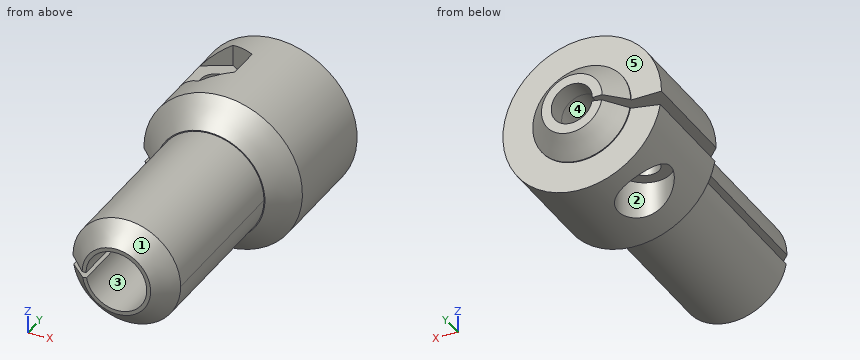
```python
from build123d import *

# Parameters (mm, degrees)
REVOLUTION_ANGLE = 350
SKETCH002_R      = 1.5
POCKET_DEPTH     = 22.101
POCKET001_DEPTH  = 9
SKETCH003_R      = 2.7
POCKET002_DEPTH  = 11
SKETCH004_R      = 8.1
SKETCH004_R_2    = 5.5
POCKET003_DEPTH  = 18
CHAMFER_SIZE     = 2.5
CHAMFER001_SIZE  = 2
PAD_DEPTH        = 2
CHAMFER002_SIZE  = 1.9


with BuildPart() as part:
    # Sketch → Revolution (revolve)
    with BuildSketch(Plane.XY):
        Polygon((-2.1, 8), (-2.1, 0), (-3.1, 0), (-3.1, -23), (-8.1, -23), (-8.1, 8), align=None)
    revolve(axis=Axis((0, 0, 0), (0, 1, 0)), revolution_arc=REVOLUTION_ANGLE)

    # Sketch002 (on DatumPlane) → Pocket (cut, through all)
    with BuildSketch(Plane.XY.offset(14)):
        with Locations((-3.8, 3.2)):
            Circle(SKETCH002_R)
    extrude(amount=-POCKET_DEPTH, mode=Mode.SUBTRACT)

    # Sketch001 (on DatumPlane) → Pocket001 (cut)
    with BuildSketch(Plane.XY.offset(14)):
        Polygon((-3.8, -0.1), (-0.942116, 1.55), (-0.942116, 4.85), (-3.8, 6.5), (-6.657884, 4.85), (-6.657884, 1.55), align=None)
    extrude(amount=-POCKET001_DEPTH, mode=Mode.SUBTRACT)

    # Sketch003 (on DatumPlane) → Pocket002 (cut)
    with BuildSketch(Plane.XY.offset(-15)):
        with Locations((-3.8, 3.2)):
            Circle(SKETCH003_R)
    extrude(amount=POCKET002_DEPTH, mode=Mode.SUBTRACT)

    # Sketch004 (on Face8 of Pocket002) → Pocket003 (cut)
    with BuildSketch(Plane.XZ.offset(23)):
        Circle(SKETCH004_R)
        Circle(SKETCH004_R_2, mode=Mode.SUBTRACT)
    extrude(amount=-POCKET003_DEPTH, mode=Mode.SUBTRACT)

    # Chamfer
    chamfer_edges = [part.edges().sort_by_distance(p)[0] for p in [
        (0.705962, -5, -8.069177),
    ]]
    chamfer(chamfer_edges, length=CHAMFER_SIZE)

    # Chamfer001
    chamfer001_edges = [part.edges().sort_by_distance(p)[0] for p in [
        (0.479357, -23, -5.479071),
    ]]
    chamfer(chamfer001_edges, length=CHAMFER001_SIZE)

    # Sketch005 (on Face10 of Chamfer001) → Pad (join)
    with BuildSketch(Plane(origin=(0, 8, 0), x_dir=(-1, 0, 0), z_dir=(0, 1, 0))):
        with BuildLine():
            ThreePointArc((5, 0), (-4.980973, 0.435779), (4.924039, -0.868241))
            Line((2.068096, -0.364661), (4.924039, -0.868241))
            ThreePointArc((2.1, 0), (-2.092009, 0.183027), (2.068096, -0.364661))
            Line((2.1, 0), (5, 0))
        make_face()
    extrude(amount=PAD_DEPTH)

    # Chamfer002
    chamfer002_edges = [part.edges().sort_by_distance(p)[0] for p in [
        (4.980973, 10, 0.435779),
    ]]
    chamfer(chamfer002_edges, length=CHAMFER002_SIZE)


solid = part.part
```
Check sheet for the modelled part. Datum: model origin and axes. Units: mm. Face numbers are marked on the shaded views. A direction names the side the tool comes from. Give positions to 0.01 mm unless a question says otherwise; leave off trailing zeros. Write each loop counter-clockwise with the first axis right and the second up, starting at its lowest first coordinate (ties: lowest second). Pieces come first, ordered by that corner, then holes. Notation, with made-up numbers: (-37.5, 24) - (-5.5, 24) arc R25 ccw to (-5.5, 60) - close; hole circle Ø9 at (-12, 63). An arc over 180 degrees is marked (long way). Answer as a JSON object with one key per item and string values. Group by question number.
1) Thickness scan on probe 1 along Z at (x, y) = (0, -17.75); probe 2 along X at (y, z) = (4, 0.75); probe 3 along Z at (x, y) = (-4.25, -6.5). Record the ranges inside material, lowest first. Write a range as from..to.
2) Access from +Z, -Z, +X, -X, +Y, -Y to the whole of each face (thin tool, end or side, straight path). Record for the marked faces 4 and 5.
3) Depth check by flat-ended pin: P1, Ø1.5, axis at x = 1, y = -7.5, coming from the +Z side; P2, Ø2.5, axis at y = 2.5, z = 6.5, coming from the -X side; P3, Ø1.6, axis at x = -3, y = 2.5, coming from the -Z side. Enter the tip coordinate at first touch or a pass-through.
4) Sectioned sample at C-C (z = 1.75). Give the number of separate pieces and of enclosed holes in the cut face, then the cut area to 3 significant figures.
5) Release check for a two-part mould opening along Y. For the marked faces 1, 2 and 3 record: pulls with the +Y half, pulls with the -Y half, needs draft (parallel to the pull), parting line crosses it, or undercut.
6) Sectioned sample at B-B (y = 3.2). Record the cut outline in (x, z), then the cut area to 3 significant figures.
Geometry results:
{
 "1": {"probe 1": "z = -5.5..-3.1, 3.1..5.5", "probe 2": "x = -8.07..-5.07, -2.53..-1.96, 1.96..8.07", "probe 3": "z = -3.49..-0.75, 0..3.49"},
 "2": {"face 4": "+Y, -Y", "face 5": "+Y"},
 "3": {"P1": "stops at z = 5.49", "P2": "stops at x = -1.46", "P3": "stops at z = -4"},
 "4": {"separate pieces": "2", "enclosed holes": "1", "area": "249 mm^2"},
 "5": {"face 1": "pulls with the -Y half", "face 2": "undercut", "face 3": "needs draft"},
 "6": {"outline": "(-8.1, 0) - (-5.3, 0) - (-5.3, 5) - (-6.37, 5) arc R8.1 ccw to start; (-7.98, -1.41) arc R8.1 ccw to (-6.5, -4.83) - (-6.5, -4) - (-5.3, -4) - (-5.3, -0.93) - close; (-2.3, -4) - (-1.1, -4) - (-1.1, -8.02) arc R8.1 ccw (long way) to (-0.94, 8.05) - (-0.94, 5) - (-2.3, 5) - (-2.3, 0) - (-2.1, 0) arc R2.1 cw (long way) to (-2.07, -0.36) - (-2.3, -0.41) - close", "area": "135 mm^2"}
}
